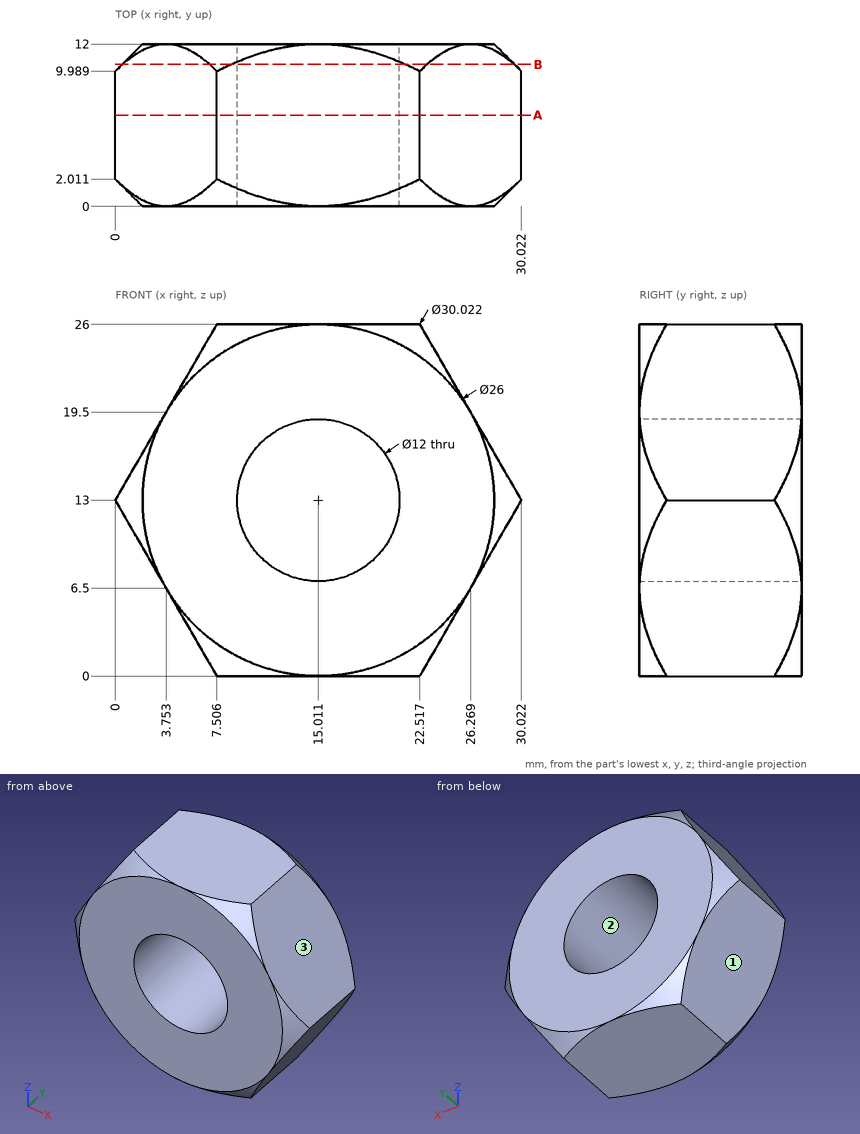
Design review of the part shown in the three views and the two pictorial views. Dimensions are in mm from the part's minimum x, y and z. Round coordinates to 2 decimals unless told otherwise and drop trailing zeros. Write each loop counter-clockwise with the first axis right and the second up, starting at its lowest first coordinate (ties: lowest second). Pieces come first, ordered by that corner, then holes. Notation, with made-up numbers: (89, 23) -> (147, 23) arc R13 ccw to (147, 39) -> close; hole circle Ø1 at (15, 29). An arc over 180 degrees is marked (long way). Use one line per item in the form item = value.
1) Mouldability with a two-part tool opening along Z and no side actions: class the marked faces 1, 2 and 3 as +Z half, -Z half, draft (parallel to the pull), parting line (faces both ways), or undercut.
Found:
face_1 = -Z half
face_2 = undercut
face_3 = +Z half
2) Take a section at A-A, the plane y = 6.75. Write out the cut boundary in (x, z) (1 decimal).
Found:
outline = (0, 13) -> (7.5, 0) -> (22.5, 0) -> (30, 13) -> (22.5, 26) -> (7.5, 26) -> close; hole circle Ø12 at (15, 13)
3) Clearance check with flat-ended pins moving along their axes: pin 1 (1.5 mm diameter, centred on y = 10, z = 18, fed in from +X); pin 2 (4 mm diameter, centred on y = 4.5, z = 5.5, fed in from +X); pin 3 (5 mm diameter, centred on x = 5, y = 1.5, fed in from -Z) (1 decimal). State where each tip first meets the part, or that it passes through.
Found:
pin_1 = 27.57
pin_2 = 26.85
pin_3 = 0.1
4) To check wall thickness, follow L1, parallel to Z at x = 13.5, y = 5.75; L2, parallel to Z at x = 15.5, y = 3; L3, parallel to X at y = 3, z = 12 (1 decimal). State the ranges of each line that lie inside material, in increasing order. Write a range as from..to.
Found:
L1 = 0..7.19, 18.81..26
L2 = 0..7.02, 18.98..26
L3 = 0.6..9.1, 20.9..29.4
5) Take a section at B-B, the plane y = 10.5. Write out the cut boundary in (x, z).
Found:
outline = (0.54, 12.06) -> (6.96, 0.94) arc R14.5 ccw to (8.59, 0) -> (21.43, 0) arc R14.5 ccw to (23.06, 0.94) -> (29.48, 12.06) arc R14.5 ccw to (29.48, 13.94) -> (23.06, 25.06) arc R14.5 ccw to (21.43, 26) -> (8.59, 26) arc R14.5 ccw to (6.96, 25.06) -> (0.54, 13.94) arc R14.5 ccw to start; hole circle Ø12 at (15.01, 13)
